Here's how the part is built. I have some questions about the finished solid (model axes, mm). A direction names the side the tool comes from. Give positions to 0.01 mm unless a question says otherwise; leave off trailing zeros. Loops run counter-clockwise (first coordinate to the right, second up) from the corner with the lowest first, then second, coordinate; pieces in that order, holes last.
Q1. If we section it at D-D (x = -65.5): Please give me the cut outline in (y, z).
Q2. If we section it at A-A (x = -34.5): Please give me the cut outline in (y, z).
Q3. If we section it at B-B (z = -49.5): Please give me the cut outline in (x, y).
Q4. We'd pull the mould along Z, two halves only. Please class faces 1 (the face through (-21.5, 1, -7)), 2 (the face through (-37, 1, -80.1)), 3 (the face through (-47.697, 0.298, -90.883)): +Z half, -Z half, draft (parallel to the pull), parting line (faces both ways), or undercut.
Q5. For faces 4 (the face through (-52.93, 1.14, -86.6)), 5 (the face through (-27, 2.25, -6)), 6 (the face through (-50.35, -2.82, -6.42)), 7 (the face through (-22.07, 1.14, -13.4)), 8 (the face through (-21.5, 1, -93)), which set-ups out of +Z, -Z, +X, -X, +Y, -Y let a thin tool reach every point of the face, with its end or its side?
Q6. Will these pins go through, and if not, where does the flat tip stop? P1, Ø0.5, axis at y = 2.5, z = -81.5, coming from the -X side; P2, Ø9, axis at x = -26.5, z = -10, coming from the +Y side; P3, Ø1.1, axis at y = 1.5, z = -8, coming from the +X side.
Q7. I need wall thicknesses on line 1 (Z direction, x = -48, y = 1); line 2 (Z direction, x = -27, y = -0.55); line 3 (Z direction, x = -31, y = 1.5). Which ranges of each line are inside material? Lowest first, please.
Q8. If we section it at C-C (x = -48): Give the number of separate pieces and of enclosed holes in the cut face, plus the area to 3 significant figures.
Autodesk Inventor part; units mm, degrees
ref_plane "YZ Plane" through (0, 0, 0) normal (1, 0, 0) x (0, 1, 0)
ref_plane "XZ Plane" through (0, 0, 0) normal (0, 1, 0) x (-1, 0, 0)
ref_plane "XY Plane" through (0, 0, 0) normal (0, 0, 1) x (1, 0, 0)
sketch "Boceto1" plane through (0, 0, 0) normal (0, 1, 0) x (-1, 0, 0)
  line L0 (0, 0) -> (75, 0)
  line L1 (75, 0) -> (75, -100)
  line L2 (75, -100) -> (0, -100)
  line L3 (0, -100) -> (0, 0)
  line L4 (7.4, -80.1) -> (67.6, -80.1)
  line L5 (67.6, -80.1) -> (67.6, -19.9)
  line L6 (67.6, -19.9) -> (7.4, -19.9)
  line L7 (7.4, -19.9) -> (7.4, -80.1)
  line L8 (7.4, -80.1) -> (67.6, -19.9) construction
  line L9 (67.6, -80.1) -> (7.4, -19.9) construction
  line L10 (70.6, -16.9) -> (70.6, -83.1)
  line L11 (70.6, -83.1) -> (4.4, -83.1)
  line L12 (4.4, -83.1) -> (4.4, -16.9)
  line L13 (4.4, -16.9) -> (70.6, -16.9)
  line L14 (53.5, -1.5) -> (21.5, -1.5)
  line L15 (21.5, -1.5) -> (21.5, -14)
  line L16 (21.5, -14) -> (53.5, -14)
  line L17 (53.5, -14) -> (53.5, -1.5)
  line L18 (67.6, -50) -> (7.4, -50) construction
  line L19 (53.5, -7.75) -> (48, -7.75) construction
  line L20 (48, -7.75) -> (27, -7.75) construction
  line L21 (27, -7.75) -> (21.5, -7.75) construction
  circle A0 centre (48, -7.75) radius 1.4
  circle A1 centre (27, -7.75) radius 1.4
  line L22 (53.5, -98.5) -> (21.5, -98.5)
  line L23 (21.5, -98.5) -> (21.5, -86)
  line L24 (21.5, -86) -> (53.5, -86)
  line L25 (53.5, -86) -> (53.5, -98.5)
  circle A2 centre (48, -92.25) radius 1.4
  circle A3 centre (27, -92.25) radius 1.4
  line L26 (58.4347, 0) -> (58.4347, -14) construction
  line L27 (68.2, -14.5) -> (75, -14.5) construction
  line L28 (37.5, -19.9) -> (37.5, -80.1) construction
  circle A4 centre (48, -92.25) radius 1.4
  line L29 (48, -7.75) -> (27, -7.75)
  line L30 (37.5, -1.5) -> (37.5, 0)
  line L31 (37.5, -1.5) -> (37.5, -50)
  point P0 (37.5, -14)
  point P1 (37.5, -16.9)
  point P2 (37.5, -98.5)
  point P3 (37.5, -100)
  dimension "d0" = 100
  dimension "d1" = 75
  dimension "d2" = 60.2
  dimension "d3" = 60.2
  dimension "d4" = 3
  dimension "d5" = 12.5
  dimension "d6" = 32
  dimension "d8" = 5.5
  dimension "d9" = 5.5
  dimension "d10" = 2.8
  dimension "d11" = 2.8
  dimension "d14" = 14
  dimension "d32" = 1.5
  dimension "d36" = 1.5
extrude "Extrusión1" add sketch "Boceto1" along normal blind 3 contours L13 L10 L11 L12
extrude "Extrusión2" add sketch "Boceto1" against normal blind 4 contours L14 L17 L16 L31 | L31 L16 L15 L14 | L0 L1 L2 L3 | L22 L23 L24 L25
extrude "Extrusión3" add sketch "Boceto1" along normal blind 2.25 contours L14 L17 L16 L31 | L31 L16 L15 L14 | L22 L23 L24 L25
sketch "Boceto2" plane through (0, 2.25, 0) normal (0, 1, 0) x (1, 0, 0)
  line L0 (-53.5, 1.5) -> (-21.5, 1.5)
  line L1 (-37.5, 1.5) -> (-37.5, 14)
  line L2 (-21.5, 14) -> (-53.5, 14)
  line L3 (-32.5, 1.5) -> (-42.5, 1.5)
  line L4 (-42.5, 1.5) -> (-42.5, 14)
  line L5 (-42.5, 14) -> (-32.5, 14)
  line L6 (-32.5, 14) -> (-32.5, 1.5)
  line L7 (-32.5, 1.5) -> (-42.5, 14) construction
  line L8 (-42.5, 1.5) -> (-32.5, 14) construction
  line L9 (-67.6, 50) -> (-7.4, 50) construction
  line L10 (-53.5, 98.5) -> (-21.5, 98.5)
  line L11 (-21.5, 86) -> (-53.5, 86)
  line L12 (-42.5, 98.5) -> (-42.5, 86)
  line L13 (-32.5, 86) -> (-32.5, 98.5)
  point P0 (0, 0)
  point P1 (-37.5, 7.75)
  point P2 (-42.5, 98.5)
  point P3 (-42.5, 1.5)
  point P4 (-32.5, 1.5)
  point P5 (-32.5, 14)
  dimension "d22" = 10
extrude "Extrusión4" cut sketch "Boceto2" against normal blind 1.1
extrude "Extrusión5" add sketch "Boceto1" against normal blind 4 contours L6 L5 L4 L7 | L13 L10 L11 L12
sketch "Boceto3" plane through (0, 3, 0) normal (0, 1, 0) x (1, 0, 0)
  line L0 (-37.5, 19.9) -> (-37.5, 80.1) construction
  line L1 (-70.6, 16.9) -> (-4.4, 16.9)
  line L2 (-37.5, 16.9) -> (-37.5, 83.1)
  line L3 (-4.4, 83.1) -> (-70.6, 83.1)
  line L4 (-37.25, 16.9) -> (-37.75, 16.9)
  line L5 (-37.75, 16.9) -> (-37.75, 83.1)
  line L6 (-37.75, 83.1) -> (-37.25, 83.1)
  line L7 (-37.25, 83.1) -> (-37.25, 16.9)
  line L8 (-37.25, 16.9) -> (-37.75, 83.1) construction
  line L9 (-37.75, 16.9) -> (-37.25, 83.1) construction
  point P0 (0, 0)
  point P1 (-37.5, 50)
  point P2 (-37.25, 16.9)
  point P3 (-37.25, 83.1)
  point P4 (-37.75, 16.9)
  dimension "d27" = 0.5
extrude "Extrusión6" cut sketch "Boceto3" against normal blind 1
sketch "Boceto4" plane through (-53.5, 0, -1.5) normal (0, 0, 1) x (1, 0, 0)
  line L0 (16.25, 2) -> (15.75, 2)
  line L1 (21, 1.15) -> (11, 1.15)
  line L2 (-21.5, 0) -> (53.5, 0)
  line L3 (15.75, 2) -> (15.75, 3)
fillet "Empalme1" radius 2 4 edges at (-53.5, 1.125, -86) (-21.5, 1.125, -86) (-21.5, 1.125, -14) (-53.5, 1.125, -14)
sketch "Boceto5" plane through (-53.5, 0, -1.5) normal (0, 0, 1) x (1, 0, 0)
  line L0 (16.25, 2) -> (15.75, 2)
  line L1 (21, 1.15) -> (11, 1.15)
  point P0 (53.5, 0)
sketch "Boceto6" plane through (0, -4, 0) normal (0, -1, 0) x (1, 0, 0)
  line L0 (-27, -7.75) -> (-21.5, -7.75) construction
  circle A0 centre (-48, -7.75) radius 1.4
  line L1 (-46.4401, -5.0506) -> (-44.8823, -7.7512)
  line L2 (-44.8823, -7.7512) -> (-46.4422, -10.4506)
  line L3 (-46.4422, -10.4506) -> (-49.5599, -10.4494)
  line L4 (-49.5599, -10.4494) -> (-51.1177, -7.7488)
  line L5 (-51.1177, -7.7488) -> (-49.5578, -5.0494)
  line L6 (-49.5578, -5.0494) -> (-46.4401, -5.0506)
  line L7 (0, 0) -> (-75, 0)
  line L8 (-37.5, 0) -> (-37.3669, -100)
  line L9 (0, -100) -> (-75, -100)
  line L10 (-75, 0) -> (-75, -100)
  line L11 (-75, -50) -> (0, -50)
  line L12 (0, -100) -> (0, 0)
  line L13 (-28.5465, -5.0268) -> (-30.0971, -7.7316)
  line L14 (-30.0971, -7.7316) -> (-28.53, -10.4268)
  line L15 (-28.53, -10.4268) -> (-25.4123, -10.4172)
  line L16 (-25.4123, -10.4172) -> (-23.8617, -7.7125)
  line L17 (-23.8617, -7.7125) -> (-25.4288, -5.0172)
  line L18 (-25.4288, -5.0172) -> (-28.5465, -5.0268)
  line L19 (-46.4401, -94.9494) -> (-44.8823, -92.2488)
  line L20 (-44.8823, -92.2488) -> (-46.4422, -89.5494)
  line L21 (-46.4422, -89.5494) -> (-49.5599, -89.5506)
  line L22 (-49.5599, -89.5506) -> (-51.1177, -92.2512)
  line L23 (-51.1177, -92.2512) -> (-49.5578, -94.9506)
  line L24 (-49.5578, -94.9506) -> (-46.4401, -94.9494)
  line L25 (-23.8617, -92.2875) -> (-25.4288, -94.9828)
  line L26 (-25.4288, -94.9828) -> (-28.5465, -94.9732)
  line L27 (-28.5465, -94.9732) -> (-30.0971, -92.2684)
  line L28 (-30.0971, -92.2684) -> (-28.53, -89.5732)
  line L29 (-28.53, -89.5732) -> (-25.4123, -89.5828)
  line L30 (-25.4123, -89.5828) -> (-23.8617, -92.2875)
  dimension "d37" = 5.4
extrude "Extrusión7" cut sketch "Boceto6" against normal blind 2.4 contours A0 | L1 L2 L3 L4 L5 L6 | L18 L17 L16 L15 L14 L13 | L24 L23 L22 L21 L20 L19 | L25 L26 L27 L28 L29 L30
equation "\"d9\" = d8"
properties part number "Molde 663FBR 1mm"
Check sheet entries:
1. outline: (-4, -100) - (0, -100) - (0, -83.1) - (3, -83.1) - (3, -80.1) - (0, -80.1) - (0, -19.9) - (3, -19.9) - (3, -16.9) - (0, -16.9) - (0, 0) - (-4, 0) - close
2. outline: (-4, -100) - (0, -100) - (0, -98.5) - (1.15, -98.5) - (1.15, -86) - (0, -86) - (0, -83.1) - (3, -83.1) - (3, -80.1) - (0, -80.1) - (0, -19.9) - (3, -19.9) - (3, -16.9) - (0, -16.9) - (0, -14) - (1.15, -14) - (1.15, -1.5) - (0, -1.5) - (0, 0) - (-4, 0) - close
3. outline: (-75, -4) - (0, -4) - (0, 0) - (-4.4, 0) - (-4.4, 3) - (-7.4, 3) - (-7.4, 0) - (-67.6, 0) - (-67.6, 3) - (-70.6, 3) - (-70.6, 0) - (-75, 0) - close
4. face 1: draft
4. face 2: undercut
4. face 3: undercut
5. face 4: -X, +Y
5. face 5: +Z, +X, -X, +Y
5. face 6: -Y
5. face 7: +X, +Y
5. face 8: -Z, +X, +Y
6. P1: stops at x = -70.6
6. P2: stops at y = 2.25
6. P3: stops at x = -21.5
7. line 1: z = -98.5 to -93.65, -90.85 to -86, -83.1 to -80.1, -19.9 to -16.9, -14 to -9.15, -6.35 to -1.5
7. line 2: z = -100 to -93.65, -90.85 to -9.15, -6.35 to 0
7. line 3: z = -98.5 to -86, -83.1 to -80.1, -19.9 to -16.9, -14 to -1.5
8. separate pieces: 3
8. enclosed holes: 0
8. area: 427 mm2
